Verification items for the finished model (mm, model axes). Give positions to 0.01 mm unless a question says otherwise; leave off trailing zeros. Order: outer loops, then holes, each group sorted by start corner. A loop starts at its lowest first (then second) coordinate and runs counter-clockwise, first axis right, second up. Notation, with made-up numbers: (5.25, -26) -> (50.25, -26) arc R26 ccw to (50.25, -7) -> close; hole circle Ø4 at (22.5, -27.75). An arc over 180 degrees is marked (long way). Return JSON: item names as keys, results as strings. Group by question number.
(1) Cross-section at A-A on z = 0. Enter the section's corners in (x, y), then the cut area to 3 significant figures.
(2) Thickness scan on line 1 along Z through (x, y) = (-54, 2.8). Record the ranges inside material, lowest first.
(3) Depth check by flat-ended pin: pin 1 Ø6 at (x, z) = (29, 35.5) entering from -Y; pin 2 Ø0.9 at (y, z) = (1, 0.5) entering from +X; pin 3 Ø0.9 at (x, y) = (-52, 1) entering from -Z. Enter the tip coordinate at first touch or a pass-through.
from build123d import *

# Parameters (mm, degrees)
SKETCH1_W           = 180
SKETCH1_H           = 180
BOSS_EXTRUDE1_DEPTH = 3
SKETCH2_W           = 5
SKETCH2_H           = 3
CUT_EXTRUDE1_DEPTH  = 3
SKETCH4_W           = 5
SKETCH4_H           = 3
CUT_EXTRUDE2_DEPTH  = 3
SKETCH5_W           = 3
SKETCH5_H           = 5
CUT_EXTRUDE3_DEPTH  = 3
SKETCH6_W           = 3
SKETCH6_H           = 5
CUT_EXTRUDE4_DEPTH  = 3
SKETCH7_W           = 10
SKETCH7_H           = 3
SKETCH7_W_2         = 3
SKETCH7_H_2         = 10
CUT_EXTRUDE5_DEPTH  = 10


with BuildPart() as part:
    # Sketch1 → Boss-Extrude1 (new body)
    with BuildSketch(Plane(origin=(0, 0, 0), x_dir=(1, 0, 0), z_dir=(0, 1, 0))):
        Rectangle(SKETCH1_W, SKETCH1_H)
    extrude(amount=BOSS_EXTRUDE1_DEPTH)

    # Sketch2 → Cut-Extrude1 (cut)
    with BuildSketch(Plane(origin=(0, 3, 0), x_dir=(1, 0, 0), z_dir=(0, 1, 0))):
        with Locations((-2.5, 88.5)):
            Rectangle(SKETCH2_W, SKETCH2_H)
        with Locations((2.5, 88.5)):
            Rectangle(SKETCH2_W, SKETCH2_H)
    extrude(amount=-CUT_EXTRUDE1_DEPTH, mode=Mode.SUBTRACT)

    # Sketch4 → Cut-Extrude2 (cut)
    with BuildSketch(Plane(origin=(0, 3, 0), x_dir=(1, 0, 0), z_dir=(0, 1, 0))):
        with Locations((-2.5, -88.5)):
            Rectangle(SKETCH4_W, SKETCH4_H)
        with Locations((2.5, -88.5)):
            Rectangle(SKETCH4_W, SKETCH4_H)
    extrude(amount=-CUT_EXTRUDE2_DEPTH, mode=Mode.SUBTRACT)

    # Sketch5 → Cut-Extrude3 (cut)
    with BuildSketch(Plane(origin=(0, 3, 0), x_dir=(1, 0, 0), z_dir=(0, 1, 0))):
        with Locations((-88.5, 2.5)):
            Rectangle(SKETCH5_W, SKETCH5_H)
        with Locations((-88.5, -2.5)):
            Rectangle(SKETCH5_W, SKETCH5_H)
    extrude(amount=-CUT_EXTRUDE3_DEPTH, mode=Mode.SUBTRACT)

    # Sketch6 → Cut-Extrude4 (cut)
    with BuildSketch(Plane(origin=(0, 3, 0), x_dir=(1, 0, 0), z_dir=(0, 1, 0))):
        with Locations((88.5, 2.5)):
            Rectangle(SKETCH6_W, SKETCH6_H)
        with Locations((88.5, -2.5)):
            Rectangle(SKETCH6_W, SKETCH6_H)
    extrude(amount=-CUT_EXTRUDE4_DEPTH, mode=Mode.SUBTRACT)

    # Sketch7 → Cut-Extrude5 (cut)
    with BuildSketch(Plane(origin=(0, 3, 0), x_dir=(1, 0, 0), z_dir=(0, 1, 0))):
        with Locations((-50, -88.5)):
            Rectangle(SKETCH7_W, SKETCH7_H)
        with Locations((50, -88.5)):
            Rectangle(SKETCH7_W, SKETCH7_H)
        with Locations((88.5, -50)):
            Rectangle(SKETCH7_W_2, SKETCH7_H_2)
        with Locations((50, 88.5)):
            Rectangle(SKETCH7_W, SKETCH7_H)
        with Locations((-88.5, -50)):
            Rectangle(SKETCH7_W_2, SKETCH7_H_2)
        with Locations((88.5, 50)):
            Rectangle(SKETCH7_W_2, SKETCH7_H_2)
        with Locations((-88.5, 50)):
            Rectangle(SKETCH7_W_2, SKETCH7_H_2)
        with Locations((-50, 88.5)):
            Rectangle(SKETCH7_W, SKETCH7_H)
    extrude(amount=-CUT_EXTRUDE5_DEPTH, mode=Mode.SUBTRACT)


solid = part.part
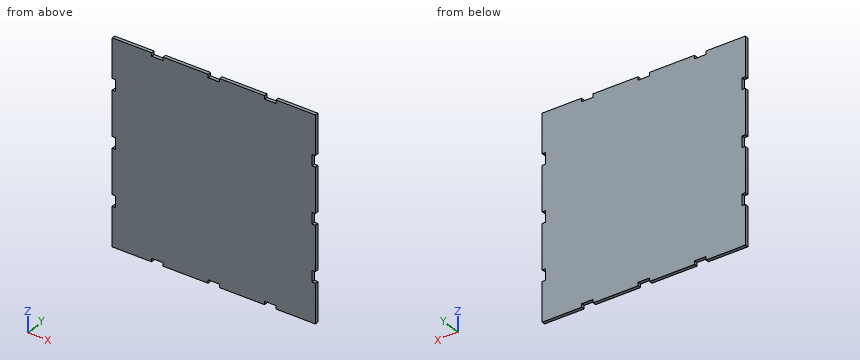
Verdict:
{
 "1": {"outline": "(-87, 0) -> (87, 0) -> (87, 3) -> (-87, 3) -> close", "area": "522 mm²"},
 "2": {"line 1": "-87 to 87"},
 "3": {"pin 1": "y = 0", "pin 2": "x = 87", "pin 3": "z = -87"}
}
